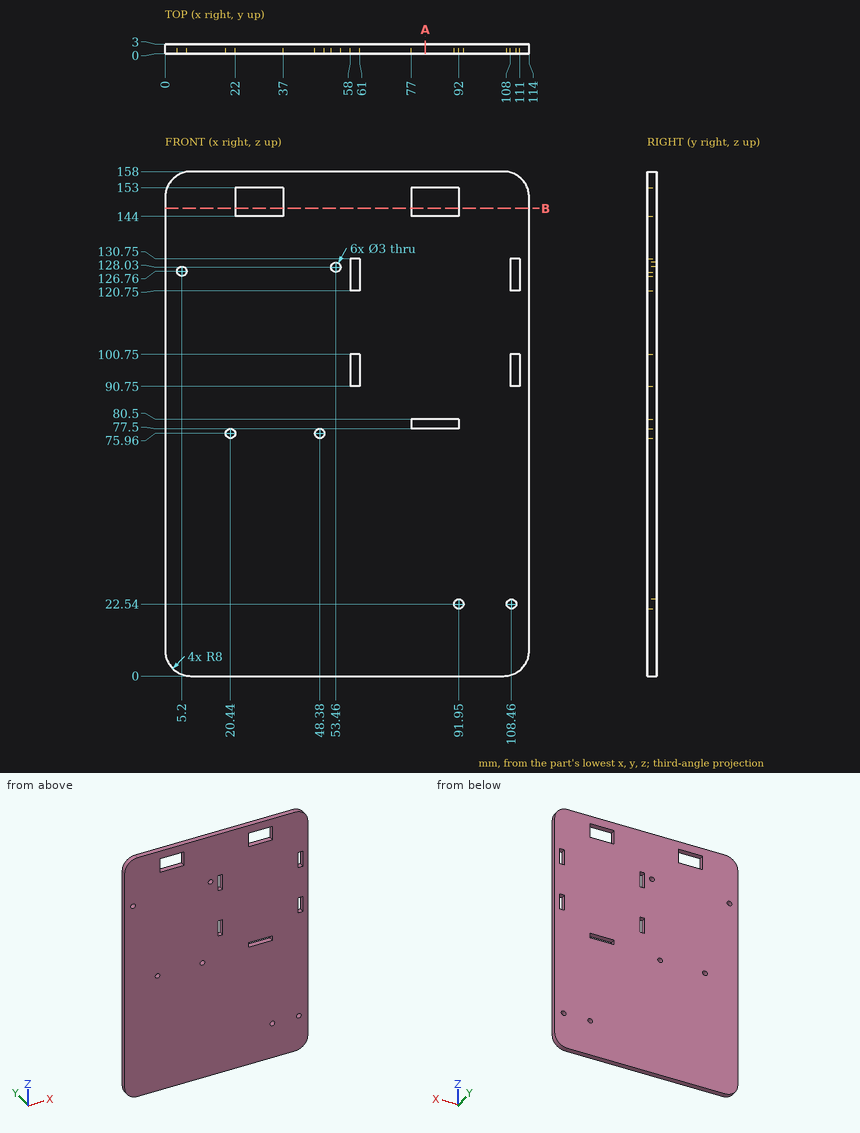
Part print with two shaded views. Sizes in mm from the minimum x, y, z corner. Coordinates: 2 decimals unless noted, no trailing zeros. Write each loop counter-clockwise with the first axis right and the second up, starting at its lowest first coordinate (ties: lowest second). Pieces come first, ordered by that corner, then holes. Notation, with made-up numbers: M 77,78 L 110,78 A32 ccw 110,116 Z; hole C -6,38 d6. An arc over 180 degrees is marked long. Return JSON: item names as keys, results as strings.
Item 1: Probe line 1 (X direction, y = 0.8, z = 22.54); line 2 (X direction, y = 1.35, z = 149); line 3 (Z direction, x = 91.95, y = 0.7). List the from-to ranges inside material, lowest first. Write a range as from..to.
Findings below:
{"line 1": "x = 0..90.45, 93.45..106.96, 109.96..114", "line 2": "x = 0..22, 37..77, 92..114", "line 3": "z = 0..21.04, 24.04..77.5, 80.5..144, 153..158"}
Item 2: Drop a flat-ended pin along its axis: pin 1 Ø0.9 at (x, y) = (109, 1) entering from +Z. Give the stop position or say it passes through.
Findings below:
{"pin 1": "stops at z = 157.58"}
Item 3: Slice it at A-A, the plane x = 81.5. Write the cut outline in (y, z).
Findings below:
{"outline": "M 0,0 L 3,0 L 3,77.5 L 0,77.5 Z; M 0,80.5 L 3,80.5 L 3,144 L 0,144 Z; M 0,153 L 3,153 L 3,158 L 0,158 Z"}
Item 4: Slice it at B-B, the plane z = 146.5. Write the cut outline in (x, y), and give its area (3 significant figures).
Findings below:
{"outline": "M 0,0 L 22,0 L 22,3 L 0,3 Z; M 37,0 L 77,0 L 77,3 L 37,3 Z; M 92,0 L 114,0 L 114,3 L 92,3 Z", "area": "252 mm2"}
